Geometry: final body of the model. Coordinates: model frame, mm. A direction names the side the tool comes from. Round coordinates to 2 decimals unless told otherwise and drop trailing zeros. Loops run counter-clockwise (first coordinate to the right, second up) from the corner with the lowest first, then second, coordinate; pieces in that order, holes last. Notation, with made-up numbers: (-14.5, 67.25) -> (17.5, 67.25) arc R33 cw to (17.5, 99.25) -> close; hole circle Ø9 at (33.25, 1). An arc over 180 degrees is marked (long way). Answer in a Markdown table with one row per item.
```python
from build123d import *

# Parameters (mm, degrees)
SKETCH1_W           = 30
SKETCH1_H           = 25
BOSS_EXTRUDE1_DEPTH = 20
SKETCH2_W           = 15
SKETCH2_H           = 25
CUT_EXTRUDE1_DEPTH  = 10
CUT_EXTRUDE2_DEPTH  = 20
CUT_EXTRUDE3_DEPTH  = 10


with BuildPart() as part:
    # Sketch1 → Boss-Extrude1 (new body)
    with BuildSketch(Plane.XY):
        with Locations((15, 12.5)):
            Rectangle(SKETCH1_W, SKETCH1_H)
    extrude(amount=BOSS_EXTRUDE1_DEPTH)

    # Sketch2 → Cut-Extrude1 (cut)
    with BuildSketch(Plane.XY.offset(20)):
        with Locations((7.5, 12.5)):
            Rectangle(SKETCH2_W, SKETCH2_H)
    extrude(amount=-CUT_EXTRUDE1_DEPTH, mode=Mode.SUBTRACT)

    # Sketch3 → Cut-Extrude2 (cut)
    with BuildSketch(Plane.ZY.offset(-15)):
        Polygon((15, 25), (20, 15), (20, 25), align=None)
    extrude(amount=-CUT_EXTRUDE2_DEPTH, mode=Mode.SUBTRACT)

    # Sketch4 → Cut-Extrude3 (cut)
    with BuildSketch(Plane(origin=(0, 25, 0), x_dir=(1, 0, 0), z_dir=(0, 1, 0))):
        Polygon((15, -10), (0, 0), (0, -10), align=None)
    extrude(amount=-CUT_EXTRUDE3_DEPTH, mode=Mode.SUBTRACT)


solid = part.part
```
Item 1: Section query D-D, the plane y = 18.25. Output: boundary loops of the cut face in (x, z) (3 decimals), and give its area (3 significant figures).
Ans:
| item | result |
|---|---|
| outline | (0, 0) -> (30, 0) -> (30, 18.375) -> (15, 18.375) -> (15, 10) -> close |
| area | 351 mm2 |
Item 2: Ray query, L1, parallel to Z at x = 2.5, y = 2.5; L2, parallel to X at y = 9.25, z = 10.25; L3, parallel to Z at x = 7, y = 23.25. Return the intervals inside material, ascending.
Ans:
| item | result |
|---|---|
| L1 | 0 to 10 |
| L2 | 15 to 30 |
| L3 | 0 to 4.67 |
Item 3: First-contact query: P1, Ø6, axis at x = 10, y = 8.5, coming from the +Z side; P2, Ø1.5, axis at y = 21, z = 6.5, coming from the -X side (3 decimals). Flat tips, straight axial feed; report the tip coordinate or a pass-through.
Ans:
| item | result |
|---|---|
| P1 | z = 10 |
| P2 | x = 8.625 |
Item 4: Section query A-A, the plane z = 2.5. Output: boundary loops of the cut face in (x, y).
Ans:
| item | result |
|---|---|
| outline | (0, 0) -> (30, 0) -> (30, 25) -> (3.75, 25) -> (3.75, 15) -> (0, 15) -> close |
Item 5: Section query C-C, the plane x = 27. Output: boundary loops of the cut face in (y, z).
Ans:
| item | result |
|---|---|
| outline | (0, 0) -> (25, 0) -> (25, 15) -> (15, 20) -> (0, 20) -> close |
Item 6: Section query B-B, the plane y = 4. Output: boundary loops of the cut face in (x, z).
Ans:
| item | result |
|---|---|
| outline | (0, 0) -> (30, 0) -> (30, 20) -> (15, 20) -> (15, 10) -> (0, 10) -> close |
Item 7: Set-up query: faces 1 (the flat face through (15, 12, 15)), 2 (the flat face through (22, 8, 20)), 3 (the flat face through (4, 15, 7)). Return all of +Z, -Z, +X, -X, +Y, -Y with unobstructed straight access to the full face (end or side cutting, diameter ignored); none if empty.
Ans:
| item | result |
|---|---|
| face 1 | +Z, -X, +Y, -Y |
| face 2 | +Z, +X, -X, +Y, -Y |
| face 3 | +Z, -X, +Y |
